from build123d import *

# Parameters (mm, degrees)
F0_W     = 76.2
F0_H     = 76.2
F1_DEPTH = 101.6
F2_SIZE2 = 101.59999
F2_SIZE  = 6.34999


# Not quite as in the source:
# - a fillet or chamfer is up to 0.001 mm smaller than in the source, because OpenCascade refuses the exact size


with BuildPart() as f1:
    # F0 (on Top) → F1 (new body)
    with BuildSketch(Plane.XY):
        with Locations((-38.1, 38.1)):
            Rectangle(F0_W, F0_H)
    extrude(amount=F1_DEPTH)

    # F2 (size 6.35 and 101.6 in the source; OpenCascade refuses exactly that, so slightly less here)
    f2_edges = [f1.edges().sort_by_distance(p)[0] for p in [
        (-38.1, 0, 101.6),
        (-76.2, 38.1, 101.6),
        (0, 38.1, 101.6),
        (-38.1, 76.2, 101.6),
    ]]
    f2_side = f1.faces().sort_by_distance((-38.1, 38.1, 101.6))[0]
    chamfer(f2_edges, length=F2_SIZE, length2=F2_SIZE2, reference=f2_side)


solid = f1.part
The model under review builds one solid part; all positions refer to its coordinate system, in mm. Round coordinates to 2 decimals unless told otherwise and drop trailing zeros. Write each loop counter-clockwise with the first axis right and the second up, starting at its lowest first coordinate (ties: lowest second). Pieces come first, ordered by that corner, then holes. Notation, with made-up numbers: M 40,12.25 L 45,12.25 A21 ccw 45,23.25 Z; hole C -19,23.25 d7. An arc over 180 degrees is marked long. Answer as CSV lines item,"result". Start each with the question number.
Q1. Wall thickness on line 1 along X through (y, z) = (28, 76.5); line 2 along Y through (x, z) = (-29.5, 72); line 3 along X through (y, z) = (67.5, 82) (3 decimals): over which ranges is each line inside the solid? List them lowest first.
Q2. Clearance check with flat-ended pins moving along their axes: P1, Ø8, axis at x = -49.5, z = 22.5, coming from the -Y side; P2, Ø12, axis at x = -39, z = 28.5, coming from the -Y side; P3, Ø1, axis at x = -65.5, z = 85.5, coming from the -Y side. State where each tip first meets the part, or that it passes through.
Q3. Consider section D-D, the plane z = 61. Give the boundary of the cut face in (x, y), then the cut area to 3 significant figures.
Q4. Consider section C-C, the plane z = 47.5. Give the boundary of the cut face in (x, y).
Result set:
1,line 1,"x = -71.42 to -4.78"
1,line 2,"y = 4.5 to 71.7"
1,line 3,"x = -71.075 to -5.125"
2,P1,"stops at y = 1.16"
2,P2,"stops at y = 1.41"
2,P3,"stops at y = 5.31"
3,outline,"M -72.39,3.81 L -3.81,3.81 L -3.81,72.39 L -72.39,72.39 Z"
3,area,"4,700 mm²"
4,outline,"M -73.23,2.97 L -2.97,2.97 L -2.97,73.23 L -73.23,73.23 Z"
